Design review of the part built by this model. Coordinates are the model's own, in mm. Face numbers are marked on the shaded views. A direction names the side the tool comes from. Coordinates: 2 decimals unless noted, no trailing zeros. Order: outer loops, then holes, each group sorted by start corner. A loop starts at its lowest first (then second) coordinate and runs counter-clockwise, first axis right, second up. Notation, with made-up numbers: M -23.75,83.5 L 5.25,83.5 A12 cw 5.25,104.5 Z; hole C 32,82 d9. An arc over 180 degrees is marked long. Use CSV: the item, a comma, the result in double quotes.
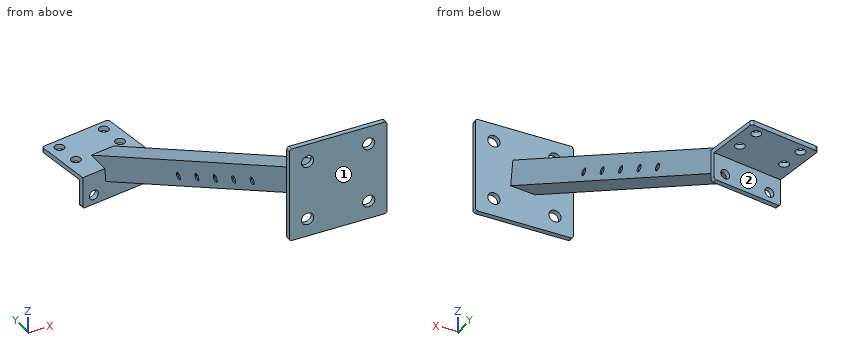
```python
from build123d import *

# Parameters (mm, degrees)
BOSS_EXTRUDE1_DEPTH      = 60
BOSS_EXTRUDE2_DEPTH      = 500
BOSS_EXTRUDE2_DEPTH_BACK = 20
CUT_EXTRUDE1_DEPTH       = 60
BOSS_EXTRUDE3_DEPTH      = 4
SKETCH7_W                = 66.53307322741853
SKETCH7_H                = 100.00000000000006
CUT_EXTRUDE2_DEPTH       = 100
CUT_EXTRUDE3_REACH       = 450.752
SKETCH8_R                = 3.999999996290614
SKETCH8_R_2              = 3.999999996290612
SKETCH8_R_3              = 3.999999996290599
SKETCH8_R_4              = 3.9999999962905974
CUT_EXTRUDE4_REACH       = 450.752
SKETCH9_R                = 4.000000002943936
SKETCH9_R_2              = 4.000000002943917
CUT_EXTRUDE5_REACH       = 492.61
SKETCH10_R               = 5.000000000000006
SKETCH10_R_2             = 5.000000000000005
FILLET1_R                = 2
FILLET2_R                = 2
SKETCH11_RX              = 3.0000000000000298
SKETCH11_RY              = 2.9901642246261853
SKETCH11_RY_2            = 2.990164224626172
SKETCH11_RX_2            = 3.000000000000057
SKETCH11_RX_3            = 3.0000000000000533
SKETCH11_RX_4            = 3.0000000000000058
SKETCH11_RY_3            = 2.9901642246261186
CUT_EXTRUDE6_DEPTH       = 450.440489599581
BODY_MOVE_COPY1_ANGLE    = 9.0000001


with BuildPart() as part:
    # Sketch1 → Boss-Extrude1 (new body)
    with BuildSketch(Plane(origin=(0, 0, 0), x_dir=(0, 0, -1), z_dir=(1, 0, 0))):
        Polygon((0, 0), (0, 50), (4, 50), (4.000000000000005, 4), (27, 4), (27, -2.82e-15), align=None)
    extrude(amount=BOSS_EXTRUDE1_DEPTH)

    # Sketch3 → Boss-Extrude2 (add, two sides: drawn at the far end of the back side and taken through both)
    with BuildSketch(Plane(origin=(0.7341522555726998, 4.014248509947268, -2.3176274578121165), x_dir=(0, -0.5000000000000011, -0.8660254037844382), z_dir=(-0.15643446504023129, -0.8553631939770857, 0.49384417029756994)).offset(-BOSS_EXTRUDE2_DEPTH_BACK)):
        Polygon((-10, 39.63065021785413), (10, 39.63065021785413), (10.000000000000002, 19.630650217854132), (-9.999999999999998, 19.630650217854132), align=None)
        Polygon((-9.000000000000002, 38.63065021785413), (9.000000000000002, 38.63065021785413), (9.000000000000005, 20.630650217854136), (-9, 20.630650217854136), align=None, mode=Mode.SUBTRACT)
    extrude(amount=BOSS_EXTRUDE2_DEPTH + BOSS_EXTRUDE2_DEPTH_BACK)

    # Sketch4 → Cut-Extrude1 (cut)
    with BuildSketch(Plane.ZY):
        Polygon((-4.000000000000005, 3.9999999999999947), (-4.000000000000005, 34.425897354185985), (-31.38403913433122, 4), align=None)
    extrude(amount=-CUT_EXTRUDE1_DEPTH, mode=Mode.SUBTRACT)

    # Sketch6 → Boss-Extrude3 (add)
    with BuildSketch(Plane(origin=(-56.75697758695906, -358.3494490271577, -6.0350178588e-07), x_dir=(0.9876883403131397, -0.15643446682069626, -2.634536772853159e-10), z_dir=(0.15643446682069626, 0.9876883403131398, 1.663381034600109e-09))):
        Polygon((60.60249934727371, -165.5937403388422), (-19.397500652726297, -165.5937403388422), (-19.397500652726286, -245.5937403388422), (60.602499347273714, -245.5937403388422), align=None)
    extrude(amount=BOSS_EXTRUDE3_DEPTH)

    # Sketch7 → Cut-Extrude2 (cut)
    with BuildSketch(Plane(origin=(-56.75697758695889, -358.34944902715785, -6.0350179691e-07), x_dir=(0.9876883403131398, -0.15643446682069573, -2.6345368210226206e-10), z_dir=(-0.15643446682069573, -0.9876883403131398, -1.6633810650131218e-09))):
        with Locations((19.033988730271286, 218.77379525877697)):
            Rectangle(SKETCH7_W, SKETCH7_H)
    extrude(amount=CUT_EXTRUDE2_DEPTH, mode=Mode.SUBTRACT)

    # Sketch8 → Cut-Extrude3 (cut, up to next)
    with BuildSketch(Plane.XY, mode=Mode.PRIVATE) as cut_extrude3_sk1:
        with Locations((10.000000000000002, 21.999999999999982)):
            Circle(SKETCH8_R)
    cut_extrude3_tool1 = extrude(cut_extrude3_sk1.sketch, amount=-CUT_EXTRUDE3_REACH, mode=Mode.PRIVATE) & part.part
    # Sketch8 → Cut-Extrude3 (cut, up to next)
    with BuildSketch(Plane.XY, mode=Mode.PRIVATE) as cut_extrude3_sk2:
        with Locations((50.00000000000001, 21.999999999999975)):
            Circle(SKETCH8_R_2)
    cut_extrude3_tool2 = extrude(cut_extrude3_sk2.sketch, amount=-CUT_EXTRUDE3_REACH, mode=Mode.PRIVATE) & part.part
    # Sketch8 → Cut-Extrude3 (cut, up to next)
    with BuildSketch(Plane.XY, mode=Mode.PRIVATE) as cut_extrude3_sk3:
        with Locations((50.00000000000001, 41.999999999999964)):
            Circle(SKETCH8_R_3)
    cut_extrude3_tool3 = extrude(cut_extrude3_sk3.sketch, amount=-CUT_EXTRUDE3_REACH, mode=Mode.PRIVATE) & part.part
    # Sketch8 → Cut-Extrude3 (cut, up to next)
    with BuildSketch(Plane.XY, mode=Mode.PRIVATE) as cut_extrude3_sk4:
        with Locations((10.000000000000009, 41.99999999999998)):
            Circle(SKETCH8_R_4)
    cut_extrude3_tool4 = extrude(cut_extrude3_sk4.sketch, amount=-CUT_EXTRUDE3_REACH, mode=Mode.PRIVATE) & part.part
    add(cut_extrude3_tool1.solids().sort_by_distance((10, 22, 0))[0], mode=Mode.SUBTRACT)
    add(cut_extrude3_tool2.solids().sort_by_distance((50, 22, 0))[0], mode=Mode.SUBTRACT)
    add(cut_extrude3_tool3.solids().sort_by_distance((50, 42, 0))[0], mode=Mode.SUBTRACT)
    add(cut_extrude3_tool4.solids().sort_by_distance((10, 42, 0))[0], mode=Mode.SUBTRACT)

    # Sketch9 → Cut-Extrude4 (cut, up to next)
    with BuildSketch(Plane.XZ, mode=Mode.PRIVATE) as cut_extrude4_sk1:
        with Locations(Location((50, -18.999999999999968, 0), (0, 0, 270))):
            Circle(SKETCH9_R)
    cut_extrude4_tool1 = extrude(cut_extrude4_sk1.sketch, amount=-CUT_EXTRUDE4_REACH, mode=Mode.PRIVATE) & part.part
    # Sketch9 → Cut-Extrude4 (cut, up to next)
    with BuildSketch(Plane.XZ, mode=Mode.PRIVATE) as cut_extrude4_sk2:
        with Locations(Location((10.000000000000002, -18.999999999999968, 0), (0, 0, 270))):
            Circle(SKETCH9_R_2)
    cut_extrude4_tool2 = extrude(cut_extrude4_sk2.sketch, amount=-CUT_EXTRUDE4_REACH, mode=Mode.PRIVATE) & part.part
    add(cut_extrude4_tool1.solids().sort_by_distance((50, 0, -19))[0], mode=Mode.SUBTRACT)
    add(cut_extrude4_tool2.solids().sort_by_distance((10, 0, -19))[0], mode=Mode.SUBTRACT)

    # Sketch10 → Cut-Extrude5 (cut, up to next)
    with BuildSketch(Plane(origin=(-56.75697758695889, -358.34944902715785, -6.0350179691e-07), x_dir=(0.9876883403131398, -0.15643446682069573, -2.6345368210226206e-10), z_dir=(-0.15643446682069573, -0.9876883403131398, -1.6633810650131218e-09)), mode=Mode.PRIVATE) as cut_extrude5_sk1:
        with Locations((-4.397500652726306, 230.59374033884228)):
            Circle(SKETCH10_R)
    cut_extrude5_tool1 = extrude(cut_extrude5_sk1.sketch, amount=-CUT_EXTRUDE5_REACH, mode=Mode.PRIVATE) & part.part
    # Sketch10 → Cut-Extrude5 (cut, up to next)
    with BuildSketch(Plane(origin=(-56.75697758695889, -358.34944902715785, -6.0350179691e-07), x_dir=(0.9876883403131398, -0.15643446682069573, -2.6345368210226206e-10), z_dir=(-0.15643446682069573, -0.9876883403131398, -1.6633810650131218e-09)), mode=Mode.PRIVATE) as cut_extrude5_sk2:
        with Locations((45.6024993472737, 230.59374033884228)):
            Circle(SKETCH10_R_2)
    cut_extrude5_tool2 = extrude(cut_extrude5_sk2.sketch, amount=-CUT_EXTRUDE5_REACH, mode=Mode.PRIVATE) & part.part
    # Sketch10 → Cut-Extrude5 (cut, up to next)
    with BuildSketch(Plane(origin=(-56.75697758695889, -358.34944902715785, -6.0350179691e-07), x_dir=(0.9876883403131398, -0.15643446682069573, -2.6345368210226206e-10), z_dir=(-0.15643446682069573, -0.9876883403131398, -1.6633810650131218e-09)), mode=Mode.PRIVATE) as cut_extrude5_sk3:
        with Locations((45.60249934727421, 180.59374033884228)):
            Circle(SKETCH10_R_2)
    cut_extrude5_tool3 = extrude(cut_extrude5_sk3.sketch, amount=-CUT_EXTRUDE5_REACH, mode=Mode.PRIVATE) & part.part
    # Sketch10 → Cut-Extrude5 (cut, up to next)
    with BuildSketch(Plane(origin=(-56.75697758695889, -358.34944902715785, -6.0350179691e-07), x_dir=(0.9876883403131398, -0.15643446682069573, -2.6345368210226206e-10), z_dir=(-0.15643446682069573, -0.9876883403131398, -1.6633810650131218e-09)), mode=Mode.PRIVATE) as cut_extrude5_sk4:
        with Locations((-4.397500652725782, 180.59374033884228)):
            Circle(SKETCH10_R)
    cut_extrude5_tool4 = extrude(cut_extrude5_sk4.sketch, amount=-CUT_EXTRUDE5_REACH, mode=Mode.PRIVATE) & part.part
    add(cut_extrude5_tool1.solids().sort_by_distance((-61.100338, -357.661529, 230.59374))[0], mode=Mode.SUBTRACT)
    add(cut_extrude5_tool2.solids().sort_by_distance((-11.715921, -365.483252, 230.59374))[0], mode=Mode.SUBTRACT)
    add(cut_extrude5_tool3.solids().sort_by_distance((-11.715921, -365.483252, 180.59374))[0], mode=Mode.SUBTRACT)
    add(cut_extrude5_tool4.solids().sort_by_distance((-61.100338, -357.661529, 180.59374))[0], mode=Mode.SUBTRACT)

    # Fillet1
    fillet1_edges = [part.edges().sort_by_distance(p)[0] for p in [
        (-75.60279387923194, -353.339634953147, 165.59373974377752),
        (-75.60279387923194, -353.3396350878763, 245.59373974377752),
        (3.412273345819247, -365.8543924335319, 245.59373972270123),
        (3.41227334581924, -365.85439229880274, 165.59373972270123),
    ]]
    fillet(fillet1_edges, radius=FILLET1_R)

    # Fillet2
    fillet2_edges = [part.edges().sort_by_distance(p)[0] for p in [
        (60, 50, -2),
        (0, 50, -2),
        (60, 1.9999999999999987, -27),
        (0, 1.9999999999999987, -27),
    ]]
    fillet(fillet2_edges, radius=FILLET2_R)

    # Sketch11 → Cut-Extrude6 (cut, through all)
    with BuildSketch(Plane(origin=(19.38896433847594, -2.659486302424582, 1.5354551326109596), x_dir=(-0.07749165674017884, 0.010629139135798351, 0.9969363392598818), z_dir=(-0.9876883405951378, 0.13547622075226887, -0.07821723252011582))):
        with Locations(Location((133.97331535443402, -240.08966554254275), (0, 0, -75.12989222147398))):
            Ellipse(SKETCH11_RX, SKETCH11_RY)
        with Locations(Location((116.69258792381987, -209.6617954111425), (0, 0, -75.12989222147398))):
            Ellipse(SKETCH11_RX, SKETCH11_RY_2)
        with Locations(Location((99.41186049320605, -179.23392527974212), (0, 0, -75.12989222147412))):
            Ellipse(SKETCH11_RX_2, SKETCH11_RY_2)
        with Locations(Location((82.13113306259201, -148.8060551483421), (0, 0, -75.12989222147439))):
            Ellipse(SKETCH11_RX_3, SKETCH11_RY_2)
        with Locations(Location((64.85040563197819, -118.37818501694186), (0, 0, -75.12989222147358))):
            Ellipse(SKETCH11_RX_4, SKETCH11_RY_3)
    extrude(amount=-CUT_EXTRUDE6_DEPTH, mode=Mode.SUBTRACT)


with BuildPart() as part_1:
    # Body-Move/Copy1: read off the stored shape, not the designer's step
    # Body-Move/Copy1: moved
    add(part.part.moved(Location((0.6987726, 367.2281966, 0))).rotate(Axis((0, 0, 0), (-1.06e-08, 0, 1.0)), BODY_MOVE_COPY1_ANGLE))


solid = part_1.part
```
(1) Clearance check with flat-ended pins moving along their axes: P1, Ø3, axis at x = -27.5, z = 69.5, coming from the -Y side; P2, Ø8, axis at x = -57, z = 187, coming from the +Y side; P3, Ø4.5, axis at x = -21, y = 1.5, coming from the -Z side; P4, Ø8, axis at x = -11.15, z = 230.59, coming from the -Y side. State where each tip first meets the part, or that it passes through.
The answers:
P1,"stops at y = 222.68"
P2,"stops at y = 4"
P3,"stops at z = 165.59"
P4,"passes through"
(2) Add section A-A on y = 299. State the section outline as (x, z) points, and give its area (3 significant figures).
The answers:
outline,"M -39.62,49.49 L -37.82,26.55 L -17.9,28.35 L -19.7,51.29 Z; hole M -38.53,48.43 L -36.91,27.79 L -18.98,29.41 L -20.6,50.05 Z"
area,"87.4 mm2"
(3) For the marked faces 1 and 2, list the 3-axis set-ups (+Z, -Z, +X, -X, +Y, -Y) from which the entire face can be reached by the end or side of a thin tool; tool diameter is ignored.
The answers:
face 1,"+Z, -Z, +X, -X, -Y"
face 2,"-Z, -X, +Y"
(4) Add section B-B on z = 22.5. State the section outline as (x, y) points, and give its area (3 significant figures).
The answers:
outline,"M -38.49,346.5 L -37.65,306.14 L -17.65,309.3 L -18.49,349.67 Z; hole M -37.45,344.64 L -36.69,308.31 L -18.69,311.16 L -19.45,347.49 Z"
area,"154 mm2"
(5) Wall thickness on probe 1 along Y at (x, z) = (-32, 214); probe 2 along Z at (x, y) = (-32.5, 131); probe 3 along Z at (x, y) = (-21, 386): over which ranges is each line inside the solid? List them lowest first.
The answers:
probe 1,"y = 0 to 4, 9.68 to 11.71"
probe 2,"z = 122.84 to 123.99, 144.77 to 145.93"
probe 3,"z = -4 to 0, 0.4 to 1.56"
